```python
from build123d import *

# Parameters (mm, degrees)
F0_R          = 31
F0_R_2        = 11.0794827648
F1_DEPTH      = 100
F2_R          = 7
F0_R_3        = 42.8779340108
F0_R_4        = 2.5
F3_DEPTH      = 10
F4_DEPTH      = 30
F5_DEPTH      = 30
F6_SIZE       = 19.99999
F7_DEPTH      = 50
F8_R          = 26.3926129655
F9_DEPTH      = 12.5
F10_S5_R      = 11.00001
F10_T6_DEPTH  = 39
F10_S11_R     = 11.00001
F10_T12_DEPTH = 39


# Not quite as in the source:
# - a fillet or chamfer that OpenCascade refuses, or shapes differently, is made with other operations: its cross-section is extruded or revolved along the edge and cut away or added
# - a fillet or chamfer is up to 0.001 mm smaller than in the source, because OpenCascade refuses the exact size


with BuildPart() as f1:
    # F0 (on Top) → F1 (new body)
    with BuildSketch(Plane.XY):
        Circle(F0_R)
        Circle(F0_R_2, mode=Mode.SUBTRACT)
        Circle(F0_R_2)
    extrude(amount=F1_DEPTH)

    # F2
    f2_edges = [f1.edges().sort_by_distance(p)[0] for p in [
        (-31, 0, 100),
    ]]
    fillet(f2_edges, radius=F2_R)

    # F0 (on Top) → F3 (join)
    with BuildSketch(Plane.XY):
        Circle(F0_R_3)
        with Locations((-25.1022907321, -25.1022907321)):
            Circle(F0_R_4, mode=Mode.SUBTRACT)
        Circle(F0_R, mode=Mode.SUBTRACT)
        with Locations((25.1022907321, 25.1022907321)):
            Circle(F0_R_4, mode=Mode.SUBTRACT)
    extrude(amount=-F3_DEPTH)

    # F0 (on Top) → F4 (join)
    with BuildSketch(Plane.XY):
        Circle(F0_R_2)
    extrude(amount=-F4_DEPTH)

    # F0 (on Top) → F5 (join)
    with BuildSketch(Plane.XY):
        Circle(F0_R)
        Circle(F0_R_2, mode=Mode.SUBTRACT)
    extrude(amount=-F5_DEPTH)

    # F6 (size 20 in the source; OpenCascade refuses exactly that, so slightly less here)
    f6_edges = [f1.edges().sort_by_distance(p)[0] for p in [
        (-31, 0, -30),
    ]]
    chamfer(f6_edges, length=F6_SIZE)

    # F7 (add): a face of the model
    f7_faces = [f1.faces().sort_by_distance(p)[0] for p in [
        (0, 0, -30),
    ]]
    extrude(f7_faces, amount=F7_DEPTH)

    # F8 (on Right) → F9 (join, symmetric)
    with BuildSketch(Plane.YZ):
        with Locations((28.3597782254, -52.3124225438)):
            Circle(F8_R)
    extrude(amount=F9_DEPTH, both=True)

    # F10: chamfer of 7 on 2 edges, made by hand


with BuildPart() as f10_tool2:
    # F10_s3 → F10_t4 (revolve)
    with BuildSketch(Plane.XY.offset(-52.3124225438)):
        Polygon((5.5, 54.7523911909), (12.5, 47.7523911909), (12.5, 54.7523911909), align=None)
    revolve(axis=Axis((12.5, 28.3597782254, -52.3124225438), (1, 0, 0)))

    # F10_s5 → F10_t6 (cut, symmetric)
    with BuildSketch(Plane.XY.offset(-52.3)):
        Circle(F10_S5_R)
    extrude(amount=F10_T6_DEPTH, both=True, mode=Mode.SUBTRACT)


with BuildPart() as f1_1:
    add(f1.part)

    # F10_t1: cut F10_tool2
    add(f10_tool2.part, mode=Mode.SUBTRACT)


with BuildPart() as f10_tool8:
    # F10_s9 → F10_t10 (revolve)
    with BuildSketch(Plane.XY.offset(-52.3124225438)):
        Polygon((-5.5, 54.7523911909), (-12.5, 47.7523911909), (-12.5, 54.7523911909), align=None)
    revolve(axis=Axis((-12.5, 28.3597782254, -52.3124225438), (1, 0, 0)))

    # F10_s11 → F10_t12 (cut, symmetric)
    with BuildSketch(Plane.XY.offset(-52.3)):
        Circle(F10_S11_R)
    extrude(amount=F10_T12_DEPTH, both=True, mode=Mode.SUBTRACT)


with BuildPart() as f1_2:
    add(f1_1.part)

    # F10_t7: cut F10_tool8
    add(f10_tool8.part, mode=Mode.SUBTRACT)


solid = f1_2.part
```
Input: part model. Units: mm. Frame: model coordinates. A direction names the side the tool comes from. Round coordinates to 2 decimals unless told otherwise and drop trailing zeros. Loops run counter-clockwise (first coordinate to the right, second up) from the corner with the lowest first, then second, coordinate; pieces in that order, holes last. Notation, with made-up numbers: M 84.25,15.5 L 142.25,15.5 A35 ccw 142.25,51.5 Z; hole C -23.5,12.5 d6. An arc over 180 degrees is marked long. Answer in a Markdown table with one row per item. Add a question column.
1. Ray query, probe 1 along X at (y, z) = (26, -61.5); probe 2 along Z at (x, y) = (-17.5, 36); probe 3 along Y at (x, z) = (-25, -7). Return the intervals inside material, ascending.
2. Set-up query: faces 1 (the face through (-12.5, 28, -52)), 2 (the face through (27.487, 25.853, -4.93)), 3 (the face through (0, -32, 0)), 4 (the face through (-2.595, -11.686, -29.029)), 5 (the face through (12.5, 28, -52)). Return all of +Z, -Z, +X, -X, +Y, -Y with unobstructed straight access to the full face (end or side cutting, diameter ignored); none if empty.
3. Mould query, pull axis Z, two halves, no side actions, for faces 6 (the face through (0.077, 54.738, -53.186)), 7 (the face through (0, 0, 100)), 8 (the face through (12.16, 47.18, -46.39)), 9 (the face through (-27.6, -25, -4.9)). Classes: released by +Z, released by -Z, zero draft, split by the parting line, or undercut.
4. Section C-C (z = 6.5). Output: boundary loops of the cut face in (x, y).
5. Contact query for flat-ended pins moving along their axis: pin 1 (6 mm diameter, centred on x = -14, z = 1, fed in from +Y); pin 2 (1.5 mm diameter, centred on x = -1.5, y = 41, fed in from -Z); pin 3 (6 mm diameter, centred on y = 7.5, z = 5.5, fed in from +X). Output: stop coordinate, or through.
Values follow:
| question | item | result |
|---|---|---|
| 1 | probe 1 | -12.5 to 12.5 |
| 1 | probe 2 | -10 to 0 |
| 1 | probe 3 | -34.84 to -27.6, -22.6 to 34.84 |
| 2 | face 1 | -Z, -X, +Y, -Y |
| 2 | face 2 | +Z, -Z |
| 2 | face 3 | +Z |
| 2 | face 4 | none |
| 2 | face 5 | -Z, +X, +Y, -Y |
| 3 | face 6 | undercut |
| 3 | face 7 | released by +Z |
| 3 | face 8 | undercut |
| 3 | face 9 | zero draft |
| 4 | outline | C 0,0 d62 |
| 5 | pin 1 | y = 41.4 |
| 5 | pin 2 | z = -75.87 |
| 5 | pin 3 | x = 30.67 |
